The model under review builds one solid part; all positions refer to its coordinate system, in mm. Face numbers are marked on the shaded views. A direction names the side the tool comes from. Coordinates: 2 decimals unless noted, no trailing zeros. Loops run counter-clockwise (first coordinate to the right, second up) from the corner with the lowest first, then second, coordinate; pieces in that order, holes last. Notation, with made-up numbers: M -38.75,21.25 L -26.75,21.25 A24 ccw -26.75,57.25 Z; hole C 41.25,22 d11. An arc over 180 degrees is marked long. Write item = value, one per line. Start each with the question number.
Q1. Wall thickness on probe 1 along X at (y, z) = (9, -3.5); probe 2 along X at (y, z) = (0.75, -39); probe 3 along X at (y, z) = (5.25, 27): over which ranges is each line inside the solid? List them lowest first.
Q2. We need section C-C on x = -11. Give the boundary of the cut face in (y, z), and give its area (3 significant figures).
Q3. Mouldability with a two-part tool opening along X and no side actions: class the marked faces 1 and 2 as released by +X, released by -X, zero draft, split by the parting line, or undercut.
Q4. For the marked faces 3 and 4, list the 3-axis set-ups (+Z, -Z, +X, -X, +Y, -Y) from which the entire face can be reached by the end or side of a thin tool; tool diameter is ignored.
Q5. We need section D-D on z = 3. Give the boundary of the cut face in (x, y).
Q6. We need section B-B on z = 28. Give the boundary of the cut face in (x, y).
Q7. Clearance check with flat-ended pins moving along their axes: pin 1 Ø10 at (y, z) = (7.5, -31) entering from +X; pin 2 Ø7.5 at (x, y) = (-39, 4.5) entering from +Z; pin 3 Ø4 at (x, z) = (-35, -15.5) entering from +Y. State where each tip first meets the part, or that it passes through.
Q8. We need section A-A on x = 38.5. Give the boundary of the cut face in (y, z), and give its area (3 significant figures).
from build123d import *

# Parameters (mm, degrees)
CROQUIS1_W                 = 69
CROQUIS1_H                 = 103
CROQUIS1_W_2               = 65
CROQUIS1_H_2               = 99
CROQUIS1_W_3               = 63
CROQUIS1_H_3               = 97
CROQUIS1_H_4               = 2
CROQUIS1_H_5               = 7
SALIENTE_EXTRUIR1_DEPTH    = 2
SALIENTE_EXTRUIR2_DEPTH    = 8
SALIENTE_EXTRUIR3_START    = -10
CROQUIS3_W                 = 69
CROQUIS3_H                 = 110
SALIENTE_EXTRUIR3_DEPTH    = 2
CROQUIS5_W                 = 12.5
CROQUIS5_H                 = 23
SALIENTE_EXTRUIR4_DEPTH    = 2
CROQUIS5_3_W               = 2
CROQUIS5_3_H               = 23
SALIENTE_EXTRUIR5_DEPTH    = 4
CORTAR_EXTRUIR1_DEPTH      = 78.24797732
CORTAR_EXTRUIR1_DEPTH_BACK = 2
CROQUIS6_R                 = 1
CROQUIS7_R                 = 4
SALIENTE_EXTRUIR6_DEPTH    = 5
CORTAR_EXTRUIR2_DEPTH      = 78.770495691
CORTAR_EXTRUIR2_DEPTH_BACK = 78.770495691
SALIENTE_EXTRUIR7_REACH    = 79.77
SALIENTE_EXTRUIR8_START    = -3
SALIENTE_EXTRUIR8_DEPTH    = 5
CORTAR_EXTRUIR3_START      = -3
CROQUIS10_3_R              = 1
CORTAR_EXTRUIR3_DEPTH      = 4


with BuildPart() as part:
    # Croquis1 → Saliente-Extruir1 (new body)
    # profile 1 of 6: a face of its own
    with BuildSketch(Plane(origin=(0, 0, 0), x_dir=(1, 0, 0), z_dir=(0, 1, 0))):
        Rectangle(CROQUIS1_W, CROQUIS1_H)
        Rectangle(CROQUIS1_W_2, CROQUIS1_H_2, mode=Mode.SUBTRACT)
    # profile 2 of 6: a face of its own
    with BuildSketch(Plane(origin=(0, 0, 0), x_dir=(1, 0, 0), z_dir=(0, 1, 0))):
        Rectangle(CROQUIS1_W_2, CROQUIS1_H_2)
        Rectangle(CROQUIS1_W_3, CROQUIS1_H_3, mode=Mode.SUBTRACT)
    # profile 3 of 6: a face of its own
    with BuildSketch(Plane(origin=(0, 0, 0), x_dir=(1, 0, 0), z_dir=(0, 1, 0))):
        Polygon((-31.5, 48.5), (31.5, 48.5), (31.5, -48.5), align=None)
    # profile 4 of 6: a face of its own
    with BuildSketch(Plane(origin=(0, 0, 0), x_dir=(1, 0, 0), z_dir=(0, 1, 0))):
        Polygon((-31.5, 48.5), (31.5, -48.5), (-31.5, -48.5), align=None)
    # profile 5 of 6: a face of its own
    with BuildSketch(Plane(origin=(0, 0, 0), x_dir=(1, 0, 0), z_dir=(0, 1, 0))):
        with Locations((0, -50.5)):
            Rectangle(CROQUIS1_W_2, CROQUIS1_H_4)
    # profile 6 of 6: a face of its own
    with BuildSketch(Plane(origin=(0, 0, 0), x_dir=(1, 0, 0), z_dir=(0, 1, 0))):
        with Locations((0, 55)):
            Rectangle(CROQUIS1_W, CROQUIS1_H_5)
    extrude(amount=-SALIENTE_EXTRUIR1_DEPTH)

    # Croquis1<3> → Saliente-Extruir2 (add)
    with BuildSketch(Plane(origin=(0, 0, 0), x_dir=(1, 0, 0), z_dir=(0, 1, 0))):
        Polygon((-32.5, -49.5), (-32.5, 49.5), (32.5, 49.5), (32.5, -49.5), (32.5, -51.5), (34.5, -51.5), (34.5, 51.5), (-34.5, 51.5), (-34.5, -51.5), (-32.5, -51.5), align=None)
    extrude(amount=SALIENTE_EXTRUIR2_DEPTH)

    # Croquis3 → Saliente-Extruir3 (add)
    with BuildSketch(Plane.XZ.offset(2).offset(SALIENTE_EXTRUIR3_START)):
        with Locations((0, -3.5)):
            Rectangle(CROQUIS3_W, CROQUIS3_H)
    extrude(amount=-SALIENTE_EXTRUIR3_DEPTH)

    # Croquis5 → Saliente-Extruir4 (add)
    with BuildSketch(Plane.XZ.offset(2)):
        with Locations((-40.75, 28)):
            Rectangle(CROQUIS5_W, CROQUIS5_H)
        with Locations((40.75, 28)):
            Rectangle(CROQUIS5_W, CROQUIS5_H)
        with Locations((40.75, -35)):
            Rectangle(CROQUIS5_W, CROQUIS5_H)
        with Locations((-40.75, -35)):
            Rectangle(CROQUIS5_W, CROQUIS5_H)
    extrude(amount=-SALIENTE_EXTRUIR4_DEPTH)

    # Croquis5<3> → Saliente-Extruir5 (add)
    with BuildSketch(Plane.XZ.offset(2)):
        with Locations((48, 28)):
            Rectangle(CROQUIS5_3_W, CROQUIS5_3_H)
        with Locations((48, -35)):
            Rectangle(CROQUIS5_3_W, CROQUIS5_3_H)
        with Locations((-48, -35)):
            Rectangle(CROQUIS5_3_W, CROQUIS5_3_H)
        with Locations((-48, 28)):
            Rectangle(CROQUIS5_3_W, CROQUIS5_3_H)
    extrude(amount=-SALIENTE_EXTRUIR5_DEPTH)

    # Croquis6 → Cortar-Extruir1 (cut, two sides: drawn at the far end of the back side and taken through both)
    with BuildSketch(Plane(origin=(0, 10, 0), x_dir=(1, 0, 0), z_dir=(0, 1, 0)).offset(-CORTAR_EXTRUIR1_DEPTH_BACK)):
        with Locations(Location((32, 3.5, 0), (0, 0, 270))):
            Circle(CROQUIS6_R)
        with Locations(Location((-32, 3.5, 0), (0, 0, 270))):
            Circle(CROQUIS6_R)
    extrude(amount=CORTAR_EXTRUIR1_DEPTH + CORTAR_EXTRUIR1_DEPTH_BACK, mode=Mode.SUBTRACT)

    # Croquis7 → Saliente-Extruir6 (add)
    with BuildSketch(Plane(origin=(0, 10, 0), x_dir=(1, 0, 0), z_dir=(0, 1, 0))):
        with Locations(Location((0, 35, 0), (0, 0, 270))):
            Circle(CROQUIS7_R)
        with Locations(Location((0, -28, 0), (0, 0, 270))):
            Circle(CROQUIS7_R)
    extrude(amount=SALIENTE_EXTRUIR6_DEPTH)

    # Croquis8 → Cortar-Extruir2 (cut, two sides: drawn at the far end of the back side and taken through both)
    with BuildSketch(Plane(origin=(0, 0, 0), x_dir=(1, 0, 0), z_dir=(0, 1, 0)).offset(-CORTAR_EXTRUIR2_DEPTH_BACK)):
        with BuildLine():
            Line((-34.5, 58.5), (-34.5, 51.5))
            ThreePointArc((-34.5, 51.5), (-17.601491564, 56.73235051), (-3.06e-07, 58.5))
            Line((-3.06e-07, 58.5), (-34.5, 58.5))
        make_face()
        with BuildLine():
            Line((34.5, 58.5), (-3.06e-07, 58.5))
            ThreePointArc((-3.06e-07, 58.5), (17.601491264, 56.732350571), (34.5, 51.5))
            Line((34.5, 51.5), (34.5, 58.5))
        make_face()
    extrude(amount=CORTAR_EXTRUIR2_DEPTH + CORTAR_EXTRUIR2_DEPTH_BACK, mode=Mode.SUBTRACT)

    # Croquis9 → Saliente-Extruir7 (add, up to next)
    with BuildSketch(Plane(origin=(0, 0, 0), x_dir=(1, 0, 0), z_dir=(0, 1, 0)), mode=Mode.PRIVATE) as saliente_extruir7_sk1:
        with BuildLine():
            Line((-34.5, 51.5), (34.5, 51.5))
            ThreePointArc((34.5, 51.5), (0, 58.5), (-34.5, 51.5))
        make_face()
    saliente_extruir7_tool1 = extrude(saliente_extruir7_sk1.sketch, amount=SALIENTE_EXTRUIR7_REACH, mode=Mode.PRIVATE) - part.part
    add(saliente_extruir7_tool1.solids().sort_by_distance((0, 0, -54.309712))[0])

    # Croquis10 → Saliente-Extruir8 (add)
    with BuildSketch(Plane.XY.offset(51.5).offset(SALIENTE_EXTRUIR8_START)):
        with BuildLine():
            Line((-38.5, 0.5), (-34.5, 0.5))
            Line((-34.5, 0.5), (-34.5, 7.5))
            Line((-34.5, 7.5), (-38.5, 7.5))
            ThreePointArc((-38.5, 7.5), (-42, 4), (-38.5, 0.5))
        make_face()
    extrude(amount=-SALIENTE_EXTRUIR8_DEPTH)

    # Croquis10<3> → Cortar-Extruir3 (cut)
    with BuildSketch(Plane.XY.offset(51.5).offset(CORTAR_EXTRUIR3_START)):
        with Locations((-38.5, 4)):
            Circle(CROQUIS10_3_R)
    extrude(amount=-CORTAR_EXTRUIR3_DEPTH, mode=Mode.SUBTRACT)


solid = part.part
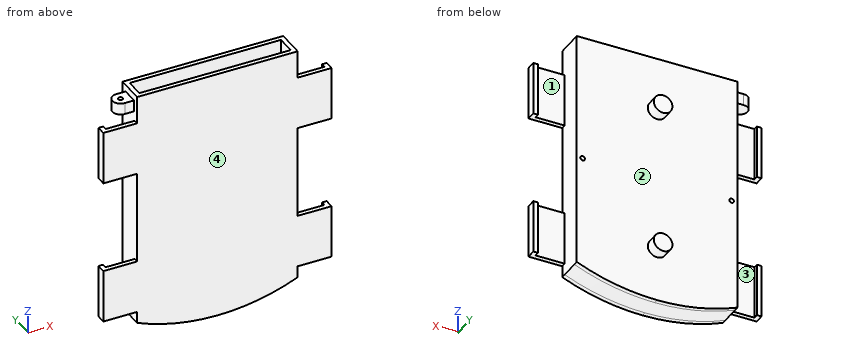
Returned:
q1.probe_1 = -34.5 to -33, -31 to 31, 33 to 34.5
q1.probe_2 = -49 to -47, -34.5 to -32.5, 32.5 to 34.5, 47 to 49
q1.probe_3 = -34.5 to -32.5, 32.5 to 34.5
q2.outline = M -2,-57.81 L 10,-57.81 L 10,51.5 L 8,51.5 L 8,-49.5 L 0,-49.5 L 0,51.5 L -2,51.5 Z
q2.area = 504 mm^2
q3.face_1 = undercut
q3.face_2 = zero draft
q4.face_3 = +Z, -Z, +Y
q4.face_4 = +Z, -Z, +X, -X, -Y
q5.outline = M -34.5,-2 L 34.5,-2 L 34.5,10 L -34.5,10 Z; hole M -32.5,0 L 32.5,0 L 32.5,8 L -32.5,8 Z
q6.outline = M -49,-2 L 49,-2 L 49,2 L 47,2 L 47,0 L 34.5,0 L 34.5,10 L 4,10 L 4,15 L -4,15 L -4,10 L -34.5,10 L -34.5,0 L -47,0 L -47,2 L -49,2 Z; hole M -32.5,0 L 32.5,0 L 32.5,8 L -32.5,8 Z
q7.pin_1 = 34.5
q7.pin_2 = 48.5
q7.pin_3 = 10
q8.outline = M -2,-46.5 L 0,-46.5 L 0,-23.5 L -2,-23.5 Z; M -2,16.5 L 0,16.5 L 0,39.5 L -2,39.5 Z
q8.area = 92.0 mm^2
